Geometry check sheet. Reference: the model listing, model coordinates, mm. A direction names the side the tool comes from. Give positions to 0.01 mm unless a question says otherwise; leave off trailing zeros. Loops run counter-clockwise (first coordinate to the right, second up) from the corner with the lowest first, then second, coordinate; pieces in that order, holes last. Notation, with made-up numbers: (65, 37.5) - (108, 37.5) arc R15 cw to (108, 55.5) - close; hole circle Ø4 at (73.25, 1). An arc over 180 degrees is marked (long way). Use a Markdown table: item, result. Add a question column.
1. Cross-section at B-B on x = 5.25. Enter the section's corners in (y, z), and give its area (3 significant figures).
2. Set-up check for faces 1 (the flat face through (4, 2, -3)), 2 (the flat face through (4, 2, -4.6)): record each of +Z, -Z, +X, -X, +Y, -Y from which the full face is reachable in a straight line by a thin tool's end or side.
3. Cross-section at A-A on z = -2. Enter the section's corners in (x, y).
4. Material ranges on L1, parallel to Z at x = 3.25, y = 1.1; L2, parallel to X at y = 2.1, z = -2.5; L3, parallel to Z at x = 7.25, y = 3, recorded low to high.
5. Depth check by flat-ended pin: P1, Ø1, axis at x = 0.5, z = -3, coming from the -Y side. Enter the tip coordinate at first touch or a pass-through.
6. Cross-section at C-C on y = 1.1. Enter the section's corners in (x, z).
from build123d import *

# Parameters (mm, degrees)
SKETCH_1_W      = 11.2
SKETCH_1_H      = 6.2
SKETCH_1_W_2    = 8
SKETCH_1_H_2    = 3
EXTRUDE_1_DEPTH = 4
FILLET_1_R      = 0.5
FILLET_2_R      = 0.5


with BuildPart() as part:
    # Эскиз1 → Бобышка-Вытянуть1 (new body)
    # profile 1 of 4: a face of its own
    with BuildSketch(Plane(origin=(0, 0, 0), x_dir=(1, 0, 0), z_dir=(0, 1, 0))):
        with Locations((4, 1.5)):
            Rectangle(SKETCH_1_W, SKETCH_1_H)
        with Locations((4, 1.5)):
            Rectangle(SKETCH_1_W_2, SKETCH_1_H_2, mode=Mode.SUBTRACT)
    # profile 2 of 4: a face of its own
    with BuildSketch(Plane(origin=(0, 0, 0), x_dir=(1, 0, 0), z_dir=(0, 1, 0))):
        Polygon((4, 4.6), (-1.6, 4.6), (-1.6, -1.6), (4, -1.6), (4, 0), (1.138545398, 0), (0, 0), (0, 1.197894344), (0, 3), (4, 3), align=None)
    # profile 3 of 4: a face of its own
    with BuildSketch(Plane(origin=(0, 0, 0), x_dir=(1, 0, 0), z_dir=(0, 1, 0))):
        Polygon((1.138545398, 0), (0, 1.197894344), (0, 0), align=None)
    # profile 4 of 4: a face of its own
    with BuildSketch(Plane(origin=(0, 0, 0), x_dir=(1, 0, 0), z_dir=(0, 1, 0))):
        Polygon((8, 0), (8, 1.197894344), (6.861454602, 0), align=None)
    extrude(amount=EXTRUDE_1_DEPTH)

    # Скругление1
    fillet_1_edges = [part.edges().sort_by_distance(p)[0] for p in [
        (8, 2, -3),
        (0, 2, -3),
    ]]
    fillet(fillet_1_edges, radius=FILLET_1_R)

    # Скругление2
    fillet_2_edges = [part.edges().sort_by_distance(p)[0] for p in [
        (9.6, 2, -4.6),
        (9.6, 2, 1.6),
        (-1.6, 2, 1.6),
        (-1.6, 2, -4.6),
        (6.861454602, 2, 0),
        (8, 2, -1.197894344),
        (0, 2, -1.197894344),
        (1.138545398, 2, 0),
    ]]
    fillet(fillet_2_edges, radius=FILLET_2_R)


solid = part.part
Values found:
| question | item | result |
|---|---|---|
| 1 | outline | (0, -4.6) - (4, -4.6) - (4, -3) - (0, -3) - close; (0, 0) - (4, 0) - (4, 1.6) - (0, 1.6) - close |
| 1 | area | 12.8 mm2 |
| 2 | face 1 | +Y, -Y |
| 2 | face 2 | -Z, +X, -X, +Y, -Y |
| 3 | outline | (-1.6, 0) - (0, 0) - (0, 4) - (-1.6, 4) - close; (8, 0) - (9.6, 0) - (9.6, 4) - (8, 4) - close |
| 4 | L1 | z = -4.6 to -3, 0 to 1.6 |
| 4 | L2 | x = -1.6 to 0, 8 to 9.6 |
| 4 | L3 | z = -4.6 to -3, -0.41 to 1.6 |
| 5 | P1 | stops at y = 0 |
| 6 | outline | (-1.6, -4.1) arc R0.5 ccw to (-1.1, -4.6) - (9.1, -4.6) arc R0.5 ccw to (9.6, -4.1) - (9.6, 1.1) arc R0.5 ccw to (9.1, 1.6) - (-1.1, 1.6) arc R0.5 ccw to (-1.6, 1.1) - close; hole (0, -2.5) arc R0.5 ccw to (0.5, -3) - (7.5, -3) arc R0.5 ccw to (8, -2.5) - (8, -1.4) arc R0.5 ccw to (7.86, -1.05) - (7.01, -0.16) arc R0.5 ccw to (6.65, 0) - (1.35, 0) arc R0.5 ccw to (0.99, -0.16) - (0.14, -1.05) arc R0.5 ccw to (0, -1.4) - close |
